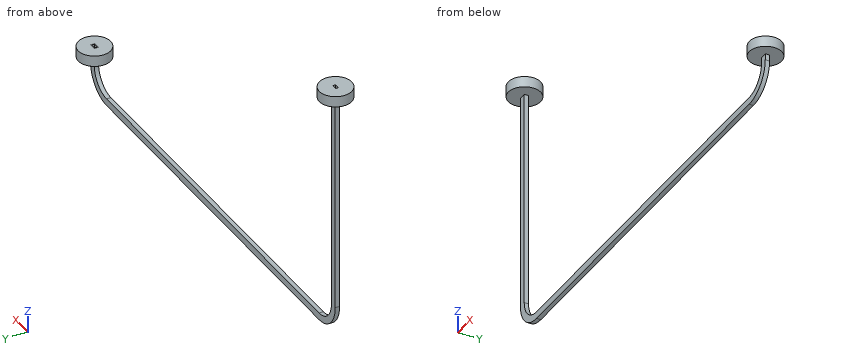
```python
from build123d import *

# Parameters (mm, degrees)
F3_W     = 4.1
F3_H     = 2.55
F3_W_2   = 3.1
F3_H_2   = 1.55
F3_R     = 9.525
F5_DEPTH = 6.35
F1_R     = 9.525
F1_W     = 4.1
F1_H     = 2.55
F6_DEPTH = 6.35


with BuildPart() as f4:
    # F4: sweep along a path in F0
    with BuildLine(Plane.XZ) as f4_path:
        Line((-260.8, 125), (-260.8, 0))
        Line((-260.8, 0), (-260.8, -10))
        ThreePointArc((-260.8, -10), (-256.289444, -20.889444), (-245.4, -25.4))
        Line((-245.4, -25.4), (-235.4, -25.4))
        Line((-235.4, -25.4), (-25.4, -25.4))
        Line((-25.4, -25.4), (-15.4, -25.4))
        ThreePointArc((-15.4, -25.4), (-4.510556, -20.889444), (0, -10))
        Line((0, -10), (0, 0))
    # F3 (on offset) → F4 (sweep)
    with BuildSketch(Plane.XY.offset(125)):
        with Locations((-260.8, 0)):
            Rectangle(F3_W, F3_H)
        with Locations((-260.8, 0)):
            Rectangle(F3_W_2, F3_H_2, mode=Mode.SUBTRACT)
    sweep(path=f4_path.line)

    # F3 (on offset) → F5 (join)
    with BuildSketch(Plane.XY.offset(125)):
        with Locations((-260.8, 0)):
            Circle(F3_R)
        with Locations((-260.8, 0)):
            Rectangle(F3_W, F3_H, mode=Mode.SUBTRACT)
    extrude(amount=-F5_DEPTH)

    # F1 (on Top) → F6 (join)
    with BuildSketch(Plane.XY):
        Circle(F1_R)
        Rectangle(F1_W, F1_H, mode=Mode.SUBTRACT)
    extrude(amount=-F6_DEPTH)


solid = f4.part
```
Design review of the part built by this model. Coordinates are the model's own, in mm. Coordinates: 2 decimals unless noted, no trailing zeros. Order: outer loops, then holes, each group sorted by start corner. A loop starts at its lowest first (then second) coordinate and runs counter-clockwise, first axis right, second up.
1) Take a section at A-A, the plane z = 39.5. Give the boundary of the cut face in (x, y) (3 decimals), and give its area (3 significant figures).
2) Clearance check with flat-ended pins moving along their axes: pin 1 (3 mm diameter, centred on y = -1, z = -8.5, fed in from -X); pin 2 (0.8 mm diameter, centred on x = -1, y = 0.5, fed in from +Z); pin 3 (0.8 mm diameter, centred on y = 0, z = 62.5, fed in from +X); pin 4 (1.5 mm diameter, centred on x = -172, y = -4, fed in from -Z). State where each tip first meets the part, or that it passes through.
3) Take a section at C-C, the plane x = -92.5. Give the boundary of the cut face in (y, z) (3 decimals).
4) Take a section at B-B, the plane y = 5.5. Give the boundary of the cut face in (x, z), and give its area (3 significant figures).
5) Wall thickness on line 1 along X through (y, z) = (0.25, -9); line 2 along X through (y, z) = (0, 92.5); line 3 along X through (y, z) = (8, -2): over which ranges is each line inside the solid? List them lowest first.
Returned:
1. outline: (-262.85, -1.275) - (-258.75, -1.275) - (-258.75, 1.275) - (-262.85, 1.275) - close; hole (-262.35, -0.775) - (-259.25, -0.775) - (-259.25, 0.775) - (-262.35, 0.775) - close
1. area: 5.65 mm2
2. pin 1: stops at x = -262.85
2. pin 2: stops at z = 0
2. pin 3: stops at x = -258.75
2. pin 4: passes through
3. outline: (-1.275, -27.45) - (1.275, -27.45) - (1.275, -23.35) - (-1.275, -23.35) - close; hole (-0.775, -26.95) - (0.775, -26.95) - (0.775, -23.85) - (-0.775, -23.85) - close
4. outline: (-268.58, 118.65) - (-253.02, 118.65) - (-253.02, 125) - (-268.58, 125) - close; (-7.78, -6.35) - (7.78, -6.35) - (7.78, 0) - (-7.78, 0) - close
4. area: 198 mm2
5. line 1: x = -262.85 to -262.35, -259.25 to -258.75, -2.05 to -1.55, 1.55 to 2.05
5. line 2: x = -262.85 to -262.35, -259.25 to -258.75
5. line 3: x = -5.17 to 5.17
